from build123d import *

# Parameters (mm, degrees)
BOX007_W               = 100
BOX007_H               = 100
BOX007_DEPTH           = 100
BOX006_W               = 100
BOX006_H               = 100
BOX006_DEPTH           = 100
BOX006_PLACEMENT_ANGLE = 90
BOX005_W               = 200
BOX005_H               = 200
BOX005_DEPTH           = 100
BOX004_W               = 20
BOX004_H               = 20
BOX004_DEPTH           = 80
BOX003_W               = 20
BOX003_H               = 20
BOX003_DEPTH           = 80
BOX002_W               = 10
BOX002_H               = 25
BOX002_DEPTH           = 35
BOX002_PITCH_ANGLE     = -15
BOX001_W               = 10
BOX001_H               = 25
BOX001_DEPTH           = 35
BOX001_PITCH_ANGLE     = 15
BOX_W                  = 20
BOX_H                  = 25
BOX_DEPTH              = 35
CYLINDER005_R          = 10
CYLINDER005_DEPTH      = 180
CYLINDER005_ROLL_ANGLE = 90
CYLINDER004_R          = 54
CYLINDER004_DEPTH      = 100
CYLINDER003_R          = 59
CYLINDER003_DEPTH      = 10
CYLINDER002_R          = 64
CYLINDER002_DEPTH      = 85
CYLINDER001_R          = 70
CYLINDER001_DEPTH      = 90
CYLINDER_R             = 80
CYLINDER_DEPTH         = 10
FILLET_R               = 3
FILLET001_R            = 5
FILLET002_R            = 5
CUT007_ROLL_ANGLE      = 90
CUT007_PITCH_ANGLE     = 45
CUT007_PLACEMENT_ANGLE = 45
CUT008_ROLL_ANGLE      = -90
CUT008_PITCH_ANGLE     = -45
CUT008_PLACEMENT_ANGLE = 45
CUT010_ROLL_ANGLE      = 90
CUT010_PITCH_ANGLE     = 45
CUT010_PLACEMENT_ANGLE = 45


with BuildPart() as cube004:
    # Box007 → Box007 (new body)
    with BuildSketch(Plane(origin=(0, 0, 0), x_dir=(-1, 0, 0), z_dir=(0, 0, 1))):
        with Locations((50, 50)):
            Rectangle(BOX007_W, BOX007_H)
    extrude(amount=BOX007_DEPTH)


with BuildPart() as cube003:
    # Box006 → Box006 (new body)
    with BuildSketch(Plane.XY):
        with Locations((50, 50)):
            Rectangle(BOX006_W, BOX006_H)
    extrude(amount=BOX006_DEPTH)


with BuildPart() as cube003_1:
    # Box006 placement: moved
    add(cube003.part.rotate(Axis((0, 0, 0), (0, 0, 1)), BOX006_PLACEMENT_ANGLE))


with BuildPart() as cube002:
    # Box005 → Box005 (new body)
    with BuildSketch(Plane(origin=(-70, -120, -100), x_dir=(1, 0, 0), z_dir=(0, 0, 1))):
        with Locations((100, 100)):
            Rectangle(BOX005_W, BOX005_H)
    extrude(amount=BOX005_DEPTH)


with BuildPart() as tab_cut_l:
    # Box004 → Box004 (new body)
    with BuildSketch(Plane(origin=(-83, -10, 20), x_dir=(1, 0, 0), z_dir=(0, 0, 1))):
        with Locations((10, 10)):
            Rectangle(BOX004_W, BOX004_H)
    extrude(amount=BOX004_DEPTH)


with BuildPart() as tab_cut_r:
    # Box003 → Box003 (new body)
    with BuildSketch(Plane(origin=(63, -10, 20), x_dir=(1, 0, 0), z_dir=(0, 0, 1))):
        with Locations((10, 10)):
            Rectangle(BOX003_W, BOX003_H)
    extrude(amount=BOX003_DEPTH)


with BuildPart() as cube001:
    # Box002 → Box002 (new body)
    with BuildSketch(Plane.XY):
        with Locations((5, 12.5)):
            Rectangle(BOX002_W, BOX002_H)
    extrude(amount=BOX002_DEPTH)


with BuildPart() as cube001_1:
    # Box002 pitch: moved
    add(cube001.part.rotate(Axis((0, 0, 0), (0, 1, 0)), BOX002_PITCH_ANGLE))


with BuildPart() as cube001_2:
    # Box002 placement: moved
    add(cube001_1.part.moved(Location((-9.95, 48, 64))))


with BuildPart() as cube:
    # Box001 → Box001 (new body)
    with BuildSketch(Plane.XY):
        with Locations((5, 12.5)):
            Rectangle(BOX001_W, BOX001_H)
    extrude(amount=BOX001_DEPTH)


with BuildPart() as cube_1:
    # Box001 pitch: moved
    add(cube.part.rotate(Axis((0, 0, 0), (0, 1, 0)), BOX001_PITCH_ANGLE))


with BuildPart() as cube_2:
    # Box001 placement: moved
    add(cube_1.part.moved(Location((0, 48, 65))))


with BuildPart() as bearing_slot:
    # Box → Box (new body)
    with BuildSketch(Plane(origin=(-10, 48, 65), x_dir=(1, 0, 0), z_dir=(0, 0, 1))):
        with Locations((10, 12.5)):
            Rectangle(BOX_W, BOX_H)
    extrude(amount=BOX_DEPTH)


with BuildPart() as bearing_holes:
    # Cylinder005 → Cylinder005 (new body)
    with BuildSketch(Plane.XY):
        Circle(CYLINDER005_R)
    extrude(amount=CYLINDER005_DEPTH)


with BuildPart() as bearing_holes_1:
    # Cylinder005 roll: moved
    add(bearing_holes.part.rotate(Axis((0, 0, 0), (1, 0, 0)), CYLINDER005_ROLL_ANGLE))


with BuildPart() as bearing_holes_2:
    # Cylinder005 placement: moved
    add(bearing_holes_1.part.moved(Location((0, 90, 65))))


with BuildPart() as through_hole:
    # Cylinder004 → Cylinder004 (new body)
    with BuildSketch(Plane.XY):
        Circle(CYLINDER004_R)
    extrude(amount=CYLINDER004_DEPTH)


with BuildPart() as inner_lip:
    # Cylinder003 → Cylinder003 (new body)
    with BuildSketch(Plane.XY.offset(80)):
        Circle(CYLINDER003_R)
    extrude(amount=CYLINDER003_DEPTH)


with BuildPart() as inner_hole:
    # Cylinder002 → Cylinder002 (new body)
    with BuildSketch(Plane.XY):
        Circle(CYLINDER002_R)
    extrude(amount=CYLINDER002_DEPTH)


with BuildPart() as body_cylinder:
    # Cylinder001 → Cylinder001 (new body)
    with BuildSketch(Plane.XY.offset(5)):
        Circle(CYLINDER001_R)
    extrude(amount=CYLINDER001_DEPTH)


with BuildPart() as cut010:
    # Cylinder → Cylinder (new body)
    with BuildSketch(Plane.XY):
        Circle(CYLINDER_R)
    extrude(amount=CYLINDER_DEPTH)

    # Fusion: union Body_Cylinder
    add(body_cylinder.part)

    # Cut: cut Inner_Hole
    add(inner_hole.part, mode=Mode.SUBTRACT)

    # Fusion001: union Inner_Lip
    add(inner_lip.part)

    # Cut001: cut Through_Hole
    add(through_hole.part, mode=Mode.SUBTRACT)

    # Fillet
    fillet_edges = [cut010.edges().sort_by_distance(p)[0] for p in [
        (-70, 0, 10),
    ]]
    fillet(fillet_edges, radius=FILLET_R)

    # Fillet001
    fillet001_edges = [cut010.edges().sort_by_distance(p)[0] for p in [
        (-80, 0, 0),
    ]]
    fillet(fillet001_edges, radius=FILLET001_R)

    # Fillet002
    fillet002_edges = [cut010.edges().sort_by_distance(p)[0] for p in [
        (-70, 0, 95),
    ]]
    fillet(fillet002_edges, radius=FILLET002_R)

    # Cut002: cut Bearing_Holes
    add(bearing_holes_2.part, mode=Mode.SUBTRACT)

    # Cut003: cut Bearing_Slot
    add(bearing_slot.part, mode=Mode.SUBTRACT)

    # Cut004: cut Cube
    add(cube_2.part, mode=Mode.SUBTRACT)

    # Cut005: cut Cube001
    add(cube001_2.part, mode=Mode.SUBTRACT)

    # Cut006: cut Tab_Cut_R
    add(tab_cut_r.part, mode=Mode.SUBTRACT)

    # Cut007: cut Tab_Cut_L
    add(tab_cut_l.part, mode=Mode.SUBTRACT)


with BuildPart() as cut010_1:
    # Cut007 roll: moved
    add(cut010.part.rotate(Axis((0, 0, 0), (1, 0, 0)), CUT007_ROLL_ANGLE))


with BuildPart() as cut010_2:
    # Cut007 pitch: moved
    add(cut010_1.part.rotate(Axis((0, 0, 0), (0, 1, 0)), CUT007_PITCH_ANGLE))


with BuildPart() as cut010_3:
    # Cut007 placement: moved
    add(cut010_2.part.rotate(Axis((0, 0, 0), (0, 0, 1)), CUT007_PLACEMENT_ANGLE))

    # Cut008: cut Cube002
    add(cube002.part, mode=Mode.SUBTRACT)


with BuildPart() as cut010_4:
    # Cut008 roll: moved
    add(cut010_3.part.rotate(Axis((0, 0, 0), (1, 0, 0)), CUT008_ROLL_ANGLE))


with BuildPart() as cut010_5:
    # Cut008 pitch: moved
    add(cut010_4.part.rotate(Axis((0, 0, 0), (0, 1, 0)), CUT008_PITCH_ANGLE))


with BuildPart() as cut010_6:
    # Cut008 placement: moved
    add(cut010_5.part.rotate(Axis((0, 0, 0), (0, 0, 1)), CUT008_PLACEMENT_ANGLE))

    # Cut009: cut Cube003
    add(cube003_1.part, mode=Mode.SUBTRACT)

    # Cut010: cut Cube004
    add(cube004.part, mode=Mode.SUBTRACT)


with BuildPart() as cut010_7:
    # Cut010 roll: moved
    add(cut010_6.part.rotate(Axis((0, 0, 0), (1, 0, 0)), CUT010_ROLL_ANGLE))


with BuildPart() as cut010_8:
    # Cut010 pitch: moved
    add(cut010_7.part.rotate(Axis((0, 0, 0), (0, 1, 0)), CUT010_PITCH_ANGLE))


with BuildPart() as cut010_9:
    # Cut010 placement: moved
    add(cut010_8.part.rotate(Axis((0, 0, 0), (0, 0, 1)), CUT010_PLACEMENT_ANGLE))


solid = cut010_9.part
Work out the finished part from the listing and answer in its coordinate system (mm). A direction names the side the tool comes from. Give positions to 0.01 mm unless a question says otherwise; leave off trailing zeros. Answer as CSV lines item,"result". Start each with the question number.
Q1. Given pin 1 Ø8 at (x, z) = (72, 23) entering from -Y; pin 2 Ø1 at (x, z) = (71.5, 39) entering from +Y; pin 3 Ø1 at (y, z) = (37, 14.5) entering from +X, each flat-ended and moving along its own axis, determine where each tip first touches the part or whether it passes through.
Q2. Find the intervals of material crossed by L1, parallel to Y at x = 91, z = 28; L2, parallel to Y at x = 61, z = 22 (3 decimals); L3, parallel to Z at x = 104, y = -21.5, in increasing order. Write a range as [from, to].
Q3. For faces 5 (the face through (56.19, 42.05, 29.65)), 6 (the face through (102.03, -18.18, 16.28)), 7 (the face through (108.38, -25.97, 13.05)), determine the directions among +Z, -Z, +X, -X, +Y, -Y from which every point of the face is accessible in a straight line to the end or side of a thin tool.
Q4. The mould has two halves that part along Y. Classify faces 1 (the face through (94.433, -18.704, 13.977)), 2 (the face through (49.018, 19.314, 48.318)), 3 (the face through (82, 13, 0)), 4 (the face through (98.565, -18.058, 15.503)): +Y half, -Y half, draft (parallel to the pull), parting line (faces both ways), or undercut.
Check result:
1,pin 1,"stops at y = 7.85"
1,pin 2,"stops at y = 11.39"
1,pin 3,"stops at x = 60.37"
2,L1,"y = [-22.51, -22.14], [-9.61, -0.27]"
2,L2,"y = [23.994, 32.979], [46.858, 47.775]"
2,L3,"z = [0, 34.7]"
3,face 5,"+Z, +X"
3,face 6,"none"
3,face 7,"+Z, -Z, +X, -Y"
4,face 1,"undercut"
4,face 2,"-Y half"
4,face 3,"draft"
4,face 4,"undercut"
